```python
from build123d import *

# Parameters (mm, degrees)
BOSS_EXTRUDE1_DEPTH                               = 2
BOSS_EXTRUDE1_DEPTH_BACK                          = 2
SKETCH1_W                                         = 48
SKETCH1_H                                         = 56.32
BOSS_EXTRUDE2_DEPTH                               = 48
SKETCH4_R                                         = 14
CUT_EXTRUDE1_DEPTH                                = 43.726478909
CSK_FOR_8_FLAT_HEAD_MACHINE_SCREW_100_D           = 4.4958
CSK_FOR_8_FLAT_HEAD_MACHINE_SCREW_100_DEPTH       = 8
CSK_FOR_8_FLAT_HEAD_MACHINE_SCREW_100_CSINK_D     = 8.4328
CSK_FOR_8_FLAT_HEAD_MACHINE_SCREW_100_CSINK_ANGLE = 100
CSK_FOR_8_FLAT_HEAD_MACHINE_SCREW_100_TIP         = 1.350674586
SKETCH13_W                                        = 33.8
SKETCH13_H                                        = 59.2
SKETCH13_W_2                                      = 25.8
SKETCH13_H_2                                      = 51.2
BOSS_EXTRUDE4_DEPTH                               = 14.76
SKETCH14_R                                        = 1
CUT_EXTRUDE5_DEPTH                                = 96.567776996


with BuildPart() as part:
    # Sketch1 → Boss-Extrude1 (new, two sides: drawn at the far end of the back side and taken through both)
    with BuildSketch(Plane.XY.offset(-BOSS_EXTRUDE1_DEPTH_BACK)):
        with Locations((0, -3.96)):
            Rectangle(SKETCH1_W, SKETCH1_H)
    extrude(amount=BOSS_EXTRUDE1_DEPTH + BOSS_EXTRUDE1_DEPTH_BACK)

    # Sketch3 → Boss-Extrude2 (add)
    with BuildSketch(Plane.ZY.offset(24)):
        Polygon((2, 24.2), (12.76, 24.2), (12.76, 18), (9.92, 18), (9.92, 20.2), (2, 20.2), align=None)
        Polygon((12.76, -18), (9.92, -18), (9.92, -28.12), (2, -28.12), (2, -32.12), (12.76, -32.12), align=None)
    extrude(amount=-BOSS_EXTRUDE2_DEPTH)

    # Sketch4 → Cut-Extrude1 (cut, through all)
    with BuildSketch(Plane(origin=(0, 0, -2), x_dir=(-1, 0, 0), z_dir=(0, 0, -1))):
        Circle(SKETCH4_R)
    extrude(amount=-CUT_EXTRUDE1_DEPTH, mode=Mode.SUBTRACT)

    # CSK for #8 Flat Head Machine Screw (100)1
    with Locations(Plane(origin=(0, -32.12, 0), x_dir=(-1, 0, 0), z_dir=(0, -1, 0))):
        with Locations((0, -5.38)):
            CounterSinkHole(CSK_FOR_8_FLAT_HEAD_MACHINE_SCREW_100_D / 2, CSK_FOR_8_FLAT_HEAD_MACHINE_SCREW_100_CSINK_D / 2, depth=CSK_FOR_8_FLAT_HEAD_MACHINE_SCREW_100_DEPTH, counter_sink_angle=CSK_FOR_8_FLAT_HEAD_MACHINE_SCREW_100_CSINK_ANGLE)
            with Locations((0, 0, -(CSK_FOR_8_FLAT_HEAD_MACHINE_SCREW_100_DEPTH + CSK_FOR_8_FLAT_HEAD_MACHINE_SCREW_100_TIP / 2))):  # 118° drill point
                Cone(0, CSK_FOR_8_FLAT_HEAD_MACHINE_SCREW_100_D / 2, CSK_FOR_8_FLAT_HEAD_MACHINE_SCREW_100_TIP, mode=Mode.SUBTRACT)

    # Sketch13 → Boss-Extrude4 (add)
    with BuildSketch(Plane.XY.offset(12.76)):
        with Locations((0, -61.72)):
            Rectangle(SKETCH13_W, SKETCH13_H)
        with Locations((0, -61.72)):
            Rectangle(SKETCH13_W_2, SKETCH13_H_2, mode=Mode.SUBTRACT)
    extrude(amount=-BOSS_EXTRUDE4_DEPTH)

    # Sketch14 → Cut-Extrude5 (cut, through all)
    with BuildSketch(Plane.XY.offset(12.76)):
        with Locations((-12.9, -36.12)):
            Circle(SKETCH14_R)
        with Locations((12.9, -36.12)):
            Circle(SKETCH14_R)
        with Locations((12.9, -87.32)):
            Circle(SKETCH14_R)
        with Locations((-12.9, -87.32)):
            Circle(SKETCH14_R)
    extrude(amount=-CUT_EXTRUDE5_DEPTH, mode=Mode.SUBTRACT)


solid = part.part
```
Build history of the part. All positions in model axes, mm. A direction names the side the tool comes from. Give positions to 0.01 mm unless a question says otherwise; leave off trailing zeros. Loops run counter-clockwise (first coordinate to the right, second up) from the corner with the lowest first, then second, coordinate; pieces in that order, holes last. Notation, with made-up numbers: (87.25, -21) -> (94.25, -21) arc R13 cw to (94.25, -7) -> close; hole circle Ø6 at (18.5, 76.25). An arc over 180 degrees is marked (long way). One line per question, with ' | ' between items.
Q1. Tool access for faces 4 (the flat face through (0, -23, 9.92)), 5 (the cylindrical face through (-0.29, -29.28, 3.15)), 6 (the flat face through (0, -36.12, 5)): list every direction of +Z, -Z, +X, -X, +Y, -Y with a clear straight run to the whole face (end or side of a thin tool).
Filled sheet:
face 4: +X, -X | face 5: none | face 6: +Z, -Z
Q2. Pull direction X, two halves, no side cores. Call faces 1 (the flat face through (16.9, -62, 5)), 2 (the flat face through (-12.9, -62, 5)), 3 (the flat face through (0, -28.12, 8)): pulls with the +X half, pulls with the -X half, needs draft (parallel to the pull), parting line crosses it, or undercut.
Filled sheet:
face 1: pulls with the +X half | face 2: undercut | face 3: needs draft
Q3. Drill centre lines: line 1 along Y through (x, z) = (-5.5, 9.75); line 2 along Y through (x, z) = (7, 10.25); line 3 along Y through (x, z) = (16, 3). Where is each one in solid material? Low to high. Write a range as [from, to].
Filled sheet:
line 1: y = [-91.32, -87.32], [-36.12, -28.12], [20.2, 24.2] | line 2: y = [-91.32, -87.32], [-36.12, -18], [18, 24.2] | line 3: y = [-91.32, -28.12], [20.2, 24.2]
Q4. Drop flat-ended pins along their axis: pin 1 (1.6 mm diameter, centred on x = 12.9, y = -36.12, fed in from -Z); pin 2 (1.5 mm diameter, centred on y = -63, z = -0.5, fed in from +X); pin 3 (5 mm diameter, centred on x = 13, y = -1.5, fed in from +Z); pin 4 (2 mm diameter, centred on y = -51, z = 10, fed in from -X). Give the stop position or say it passes through.
Filled sheet:
pin 1: passes through | pin 2: stops at x = 16.9 | pin 3: stops at z = 2 | pin 4: stops at x = -16.9
Q5. Cut at B-B, the plane x = 0. Write the cut outline in (y, z).
Filled sheet:
outline: (-91.32, -2) -> (-87.32, -2) -> (-87.32, 12.76) -> (-91.32, 12.76) -> close; (-36.12, -2) -> (-14, -2) -> (-14, 2) -> (-28.12, 2) -> (-28.12, 3.13) -> (-30.47, 3.13) -> (-32.12, 1.16) -> (-32.12, 9.6) -> (-30.47, 7.63) -> (-28.12, 7.63) -> (-28.12, 9.92) -> (-18, 9.92) -> (-18, 12.76) -> (-36.12, 12.76) -> close; (14, -2) -> (24.2, -2) -> (24.2, 12.76) -> (18, 12.76) -> (18, 9.92) -> (20.2, 9.92) -> (20.2, 2) -> (14, 2) -> close
Q6. Cut at A-A, the plane z = 5.38. Write the cut outline in (x, y).
Filled sheet:
outline: (-24, -32.12) -> (-16.9, -32.12) -> (-16.9, -91.32) -> (16.9, -91.32) -> (16.9, -32.12) -> (24, -32.12) -> (24, -28.12) -> (2.25, -28.12) -> (2.25, -30.47) -> (4.22, -32.12) -> (-4.22, -32.12) -> (-2.25, -30.47) -> (-2.25, -28.12) -> (-24, -28.12) -> close; (-24, 20.2) -> (24, 20.2) -> (24, 24.2) -> (-24, 24.2) -> close; hole (-12.9, -86.32) arc R1 ccw (long way) to (-11.9, -87.32) -> (11.9, -87.32) arc R1 ccw (long way) to (12.9, -86.32) -> (12.9, -37.12) arc R1 ccw (long way) to (11.9, -36.12) -> (-11.9, -36.12) arc R1 ccw (long way) to (-12.9, -37.12) -> close
Q7. Cut at D-D, the plane x = 18. Write the cut outline in (y, z), plus the area to 3 significant figures.
Filled sheet:
outline: (-32.12, -2) -> (24.2, -2) -> (24.2, 12.76) -> (18, 12.76) -> (18, 9.92) -> (20.2, 9.92) -> (20.2, 2) -> (-28.12, 2) -> (-28.12, 9.92) -> (-18, 9.92) -> (-18, 12.76) -> (-32.12, 12.76) -> close | area: 346 mm²
Q8. Cut at C-C, the plane y = -70.5. Write the cut outline in (x, z).
Filled sheet:
outline: (-16.9, -2) -> (-12.9, -2) -> (-12.9, 12.76) -> (-16.9, 12.76) -> close; (12.9, -2) -> (16.9, -2) -> (16.9, 12.76) -> (12.9, 12.76) -> close
